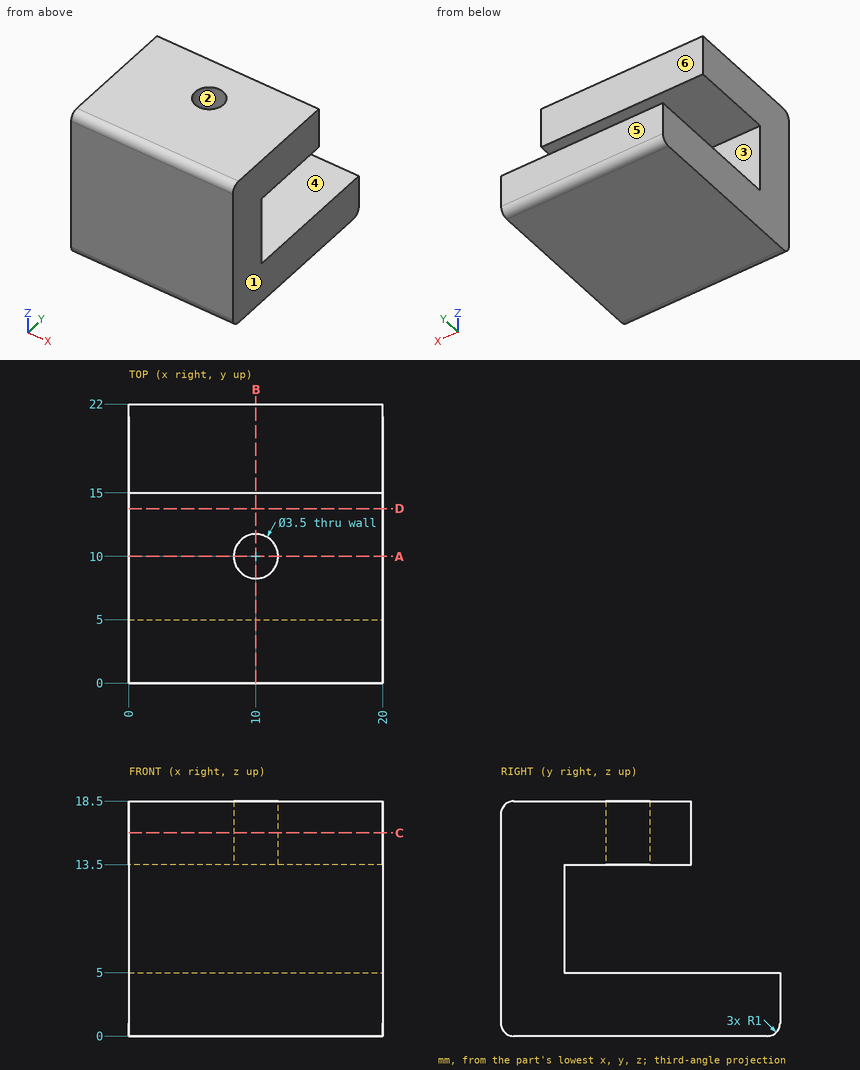
Study the drawing (mm; zero at the part's minimum x, y, z) and answer. A direction names the side the tool comes from. Round coordinates to 2 decimals unless told otherwise and drop trailing zeros. Write each loop counter-clockwise with the first axis right and the second up, starting at its lowest first coordinate (ties: lowest second). Pieces come first, ordered by that corner, then holes. Notation, with made-up numbers: (2.25, 18.25) - (42.25, 18.25) arc R36 cw to (42.25, 56.25) - close; hole circle Ø5 at (75.25, 60.5). An arc over 180 degrees is marked (long way). Use CSV: the item, a comma, the result in double quotes.
Q1. Find section B-B, the plane x = 10. Write down the section's boundary in (y, z).
Values:
outline,"(0, 1) arc R1 ccw to (1, 0) - (21, 0) arc R1 ccw to (22, 1) - (22, 5) - (5, 5) - (5, 13.5) - (8.25, 13.5) - (8.25, 18.5) - (1, 18.5) arc R1 ccw to (0, 17.5) - close; (11.75, 13.5) - (15, 13.5) - (15, 18.5) - (11.75, 18.5) - close"
Q2. Determine the mould class of the marked faces 1, 2 and 3 for opening direction Y: +Y half, -Y half, draft (parallel to the pull), parting line (faces both ways), or undercut.
Values:
face 1,"draft"
face 2,"undercut"
face 3,"+Y half"
Q3. Each of these flat-tipped pins is pushed along its axis until it touches: pin 1 Ø4 at (x, z) = (9, 10.5) entering from +Y; pin 2 Ø4 at (x, z) = (10, 16.5) entering from +Y. Where does it stop, or does it pass through?
Values:
pin 1,"stops at y = 5"
pin 2,"stops at y = 15"
Q4. Find section A-A, the plane y = 10. Write down the section's boundary in (x, z), then the cut area to 4 significant figures.
Values:
outline,"(0, 0) - (20, 0) - (20, 5) - (0, 5) - close; (0, 13.5) - (8.25, 13.5) - (8.25, 18.5) - (0, 18.5) - close; (11.75, 13.5) - (20, 13.5) - (20, 18.5) - (11.75, 18.5) - close"
area,"182.5 mm²"
Q5. A tool of negligible diameter and unlimited length cuts with its end or side. For the marked faces 4, 5 and 6, from which of +Z, -Z, +X, -X, +Y, -Y can it reach the whole face along a straight path? Write none if from no direction.
Values:
face 4,"+X, -X, +Y"
face 5,"+Z, -Z, +X, -X, +Y"
face 6,"+Z, +X, -X, +Y"
Q6. Find section D-D, the plane y = 13.75. Write down the section's boundary in (x, z), then the cut area to 3 significant figures.
Values:
outline,"(0, 0) - (20, 0) - (20, 5) - (0, 5) - close; (0, 13.5) - (20, 13.5) - (20, 18.5) - (0, 18.5) - close"
area,"200 mm²"
Q7. Find section C-C, the plane z = 16. Write down the section's boundary in (x, y).
Values:
outline,"(0, 0) - (20, 0) - (20, 15) - (0, 15) - close; hole circle Ø3.5 at (10, 10)"
Q8. Straight lines are drawn through the part: line 1 along Z through (x, y) = (18.75, 9); line 2 along Y through (x, z) = (10, 14.8); line 3 along Z through (x, y) = (12.5, 18). For each, find the intervals that lie inside material, in ascending order.
Values:
line 1,"z = 0 to 5, 13.5 to 18.5"
line 2,"y = 0 to 8.25, 11.75 to 15"
line 3,"z = 0 to 5"
